Check sheet for the modelled part. Datum: model origin and axes. Units: mm. Face numbers are marked on the shaded views. A direction names the side the tool comes from. Coordinates: 2 decimals unless noted, no trailing zeros. Write each loop counter-clockwise with the first axis right and the second up, starting at its lowest first coordinate (ties: lowest second). Pieces come first, ordered by that corner, then holes. Notation, with made-up numbers: (-22, -16) -> (13, -16) arc R19 ccw to (13, 11) -> close; hole circle Ø3 at (63, 21). An arc over 180 degrees is marked (long way). Put each result on its own line as item: value.
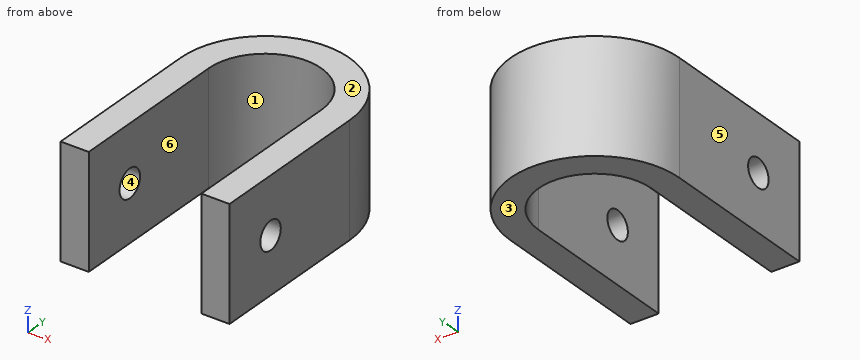
```python
from build123d import *

# Parameters (mm, degrees)
BOSS_EXTRUDE1_DEPTH = 8
SKETCH2_R           = 1
CUT_EXTRUDE1_DEPTH  = 19.572175383


with BuildPart() as part:
    # Sketch1 → Boss-Extrude1 (new body)
    with BuildSketch(Plane.XY):
        with BuildLine():
            Line((-4, 0), (-4, -11.701525476))
            Line((-4, -11.701525476), (-6, -11.701525476))
            Line((-6, -11.701525476), (-6, 0))
            ThreePointArc((-6, 0), (0, 6), (6, 0))
            Line((6, 0), (6, -11.701525476))
            Line((6, -11.701525476), (3.999999999, -11.701525476))
            Line((3.999999999, -11.701525476), (4, 0))
            ThreePointArc((4, 0), (0, 4), (-4, 0))
        make_face()
    extrude(amount=BOSS_EXTRUDE1_DEPTH)

    # Sketch2 → Cut-Extrude1 (cut, through all)
    with BuildSketch(Plane.ZY.offset(6)):
        with Locations((4, -7.701525476)):
            Circle(SKETCH2_R)
    extrude(amount=-CUT_EXTRUDE1_DEPTH, mode=Mode.SUBTRACT)


solid = part.part
```
Q1. Cross-section at D-D (z = 7). Record the cut outline in (x, y).
Recorded:
outline: (-6, -11.7) -> (-4, -11.7) -> (-4, 0) arc R4 cw to (4, 0) -> (4, -11.7) -> (6, -11.7) -> (6, 0) arc R6 ccw to (-6, 0) -> close
Q2. Cross-section at C-C (y = -7). Record the cut outline in (x, z), plus the area to 3 significant figures.
Recorded:
outline: (-6, 0) -> (-4, 0) -> (-4, 3.29) -> (-6, 3.29) -> close; (-6, 4.71) -> (-4, 4.71) -> (-4, 8) -> (-6, 8) -> close; (4, 0) -> (6, 0) -> (6, 3.29) -> (4, 3.29) -> close; (4, 4.71) -> (6, 4.71) -> (6, 8) -> (4, 8) -> close
area: 26.3 mm2
Q3. Tool access check on the marked faces 5 and 6. Record the directions out of +Z, -Z, +X, -X, +Y, -Y that give a thin tool (end or side, any length) a straight path to the whole face; none if there is none.
Recorded:
face 5: +Z, -Z, -X, +Y, -Y
face 6: +Z, -Z, -Y
Q4. Material ranges on line 1 along X through (y, z) = (-8.75, 4); line 2 along X through (y, z) = (2.25, 5.75); line 3 along Y through (x, z) = (5.25, 4), recorded low to high.
Recorded:
line 1: x = -6 to -4, 4 to 6
line 2: x = -5.56 to -3.31, 3.31 to 5.56
line 3: y = -11.7 to -8.7, -6.7 to 2.9
Q5. Cross-section at A-A (z = 4). Record the cut outline in (x, y).
Recorded:
outline: (-6, -11.7) -> (-4, -11.7) -> (-4, -8.7) -> (-6, -8.7) -> close; (-6, -6.7) -> (-4, -6.7) -> (-4, 0) arc R4 cw to (4, 0) -> (4, -6.7) -> (6, -6.7) -> (6, 0) arc R6 ccw to (-6, 0) -> close; (4, -11.7) -> (6, -11.7) -> (6, -8.7) -> (4, -8.7) -> close
Q6. Depth check by flat-ended pin: P1, Ø2.5, axis at y = -7.7, z = 4, coming from the -X side. Enter the tip coordinate at first touch or a pass-through.
Recorded:
P1: stops at x = -6
Q7. Cross-section at B-B (y = -10). Record the cut outline in (x, z).
Recorded:
outline: (-6, 0) -> (-4, 0) -> (-4, 8) -> (-6, 8) -> close; (4, 0) -> (6, 0) -> (6, 8) -> (4, 8) -> close
Q8. Mould release check, pull along Z, two halves, no side actions. Record for the marked faces 1, 2, 3 and 4: released by +Z, released by -Z, zero draft, split by the parting line, or undercut.
Recorded:
face 1: zero draft
face 2: released by +Z
face 3: released by -Z
face 4: undercut
